```python
from build123d import *

# Parameters (mm, degrees)
SKETCH1_W                = 170
SKETCH1_H                = 45
BOSS_EXTRUDE1_DEPTH      = 3
SKETCH2_W                = 6
SKETCH2_H                = 3
BOSS_EXTRUDE2_DEPTH      = 3
LPATTERN1_COUNT          = 7
LPATTERN1_PITCH          = 12
LPATTERN1_COL_COUNT      = 8
LPATTERN1_COL_PITCH      = 12
SKETCH3_W                = 6
SKETCH3_H                = 3
BOSS_EXTRUDE3_DEPTH      = 3
LPATTERN2_COUNT          = 2
LPATTERN2_PITCH          = 12
LPATTERN2_COL_COUNT      = 3
LPATTERN2_COL_PITCH      = 12
MIRROR1_COPY_1_SKETCH_W  = 6
MIRROR1_COPY_1_SKETCH_H  = 3
MIRROR1_COPY_1_DEPTH     = 3
MIRROR1_COPY_2_SKETCH_W  = 6
MIRROR1_COPY_2_SKETCH_H  = 3
MIRROR1_COPY_2_DEPTH     = 3
MIRROR1_COPY_3_SKETCH_W  = 6
MIRROR1_COPY_3_SKETCH_H  = 3
MIRROR1_COPY_3_DEPTH     = 3
MIRROR1_COPY_4_SKETCH_W  = 6
MIRROR1_COPY_4_SKETCH_H  = 3
MIRROR1_COPY_4_DEPTH     = 3
MIRROR1_COPY_5_SKETCH_W  = 6
MIRROR1_COPY_5_SKETCH_H  = 3
MIRROR1_COPY_5_DEPTH     = 3
MIRROR1_COPY_6_SKETCH_W  = 6
MIRROR1_COPY_6_SKETCH_H  = 3
MIRROR1_COPY_6_DEPTH     = 3
MIRROR1_COPY_7_SKETCH_W  = 6
MIRROR1_COPY_7_SKETCH_H  = 3
MIRROR1_COPY_7_DEPTH     = 3
MIRROR1_COPY_8_SKETCH_W  = 6
MIRROR1_COPY_8_SKETCH_H  = 3
MIRROR1_COPY_8_DEPTH     = 3
MIRROR1_COPY_9_SKETCH_W  = 6
MIRROR1_COPY_9_SKETCH_H  = 3
MIRROR1_COPY_9_DEPTH     = 3
MIRROR1_COPY_10_SKETCH_W = 6
MIRROR1_COPY_10_SKETCH_H = 3
MIRROR1_COPY_10_DEPTH    = 3
MIRROR1_COPY_11_SKETCH_W = 6
MIRROR1_COPY_11_SKETCH_H = 3
MIRROR1_COPY_11_DEPTH    = 3
MIRROR1_COPY_12_SKETCH_W = 6
MIRROR1_COPY_12_SKETCH_H = 3
MIRROR1_COPY_12_DEPTH    = 3
MIRROR1_COPY_13_SKETCH_W = 6
MIRROR1_COPY_13_SKETCH_H = 3
MIRROR1_COPY_13_DEPTH    = 3
MIRROR2_COPY_1_SKETCH_W  = 6
MIRROR2_COPY_1_SKETCH_H  = 3
MIRROR2_COPY_1_DEPTH     = 3
MIRROR2_COPY_2_SKETCH_W  = 6
MIRROR2_COPY_2_SKETCH_H  = 3
MIRROR2_COPY_2_DEPTH     = 3
MIRROR2_COPY_3_SKETCH_W  = 6
MIRROR2_COPY_3_SKETCH_H  = 3
MIRROR2_COPY_3_DEPTH     = 3


with BuildPart() as part:
    # Sketch1 → Boss-Extrude1 (new body)
    with BuildSketch(Plane(origin=(0, 0, 0), x_dir=(1, 0, 0), z_dir=(0, 1, 0))):
        Rectangle(SKETCH1_W, SKETCH1_H)
    extrude(amount=BOSS_EXTRUDE1_DEPTH)

    # Sketch2 → Boss-Extrude2 (add)
    with BuildSketch(Plane.XY.offset(22.5)):
        with Locations((6, 1.5)):
            Rectangle(SKETCH2_W, SKETCH2_H)
    boss_extrude2 = extrude(amount=BOSS_EXTRUDE2_DEPTH)

    # LPattern1: Boss-Extrude2 ×7
    with Locations(*[(i * LPATTERN1_PITCH, 0, 0) for i in range(1, LPATTERN1_COUNT)]):
        add(boss_extrude2)

    # LPattern1 col: Boss-Extrude2 ×8
    with Locations(*[(-i * LPATTERN1_COL_PITCH, 0, 0) for i in range(1, LPATTERN1_COL_COUNT)]):
        add(boss_extrude2)

    # Sketch3 → Boss-Extrude3 (add)
    with BuildSketch(Plane(origin=(85, 0, 0), x_dir=(0, 0, -1), z_dir=(1, 0, 0))):
        with Locations((6, 1.5)):
            Rectangle(SKETCH3_W, SKETCH3_H)
    boss_extrude3 = extrude(amount=BOSS_EXTRUDE3_DEPTH)

    # LPattern2: Boss-Extrude3 ×2
    with Locations(*[(0, 0, -i * LPATTERN2_PITCH) for i in range(1, LPATTERN2_COUNT)]):
        add(boss_extrude3)

    # LPattern2 col: Boss-Extrude3 ×3
    with Locations(*[(0, 0, i * LPATTERN2_COL_PITCH) for i in range(1, LPATTERN2_COL_COUNT)]):
        add(boss_extrude3)

    # Mirror1: Boss-Extrude2 across plane
    add(boss_extrude2.mirror(Plane(origin=(0, 0, 0), x_dir=(1, 0, 0), z_dir=(0, 0, -1))))

    # Mirror1 copy 1 sketch → Mirror1 copy 1 (add)
    with BuildSketch(Plane(origin=(12, 0, -22.5), x_dir=(1, 0, 0), z_dir=(0, 0, -1))):
        with Locations((6, -1.5)):
            Rectangle(MIRROR1_COPY_1_SKETCH_W, MIRROR1_COPY_1_SKETCH_H)
    extrude(amount=MIRROR1_COPY_1_DEPTH)

    # Mirror1 copy 2 sketch → Mirror1 copy 2 (add)
    with BuildSketch(Plane(origin=(24, 0, -22.5), x_dir=(1, 0, 0), z_dir=(0, 0, -1))):
        with Locations((6, -1.5)):
            Rectangle(MIRROR1_COPY_2_SKETCH_W, MIRROR1_COPY_2_SKETCH_H)
    extrude(amount=MIRROR1_COPY_2_DEPTH)

    # Mirror1 copy 3 sketch → Mirror1 copy 3 (add)
    with BuildSketch(Plane(origin=(36, 0, -22.5), x_dir=(1, 0, 0), z_dir=(0, 0, -1))):
        with Locations((6, -1.5)):
            Rectangle(MIRROR1_COPY_3_SKETCH_W, MIRROR1_COPY_3_SKETCH_H)
    extrude(amount=MIRROR1_COPY_3_DEPTH)

    # Mirror1 copy 4 sketch → Mirror1 copy 4 (add)
    with BuildSketch(Plane(origin=(48, 0, -22.5), x_dir=(1, 0, 0), z_dir=(0, 0, -1))):
        with Locations((6, -1.5)):
            Rectangle(MIRROR1_COPY_4_SKETCH_W, MIRROR1_COPY_4_SKETCH_H)
    extrude(amount=MIRROR1_COPY_4_DEPTH)

    # Mirror1 copy 5 sketch → Mirror1 copy 5 (add)
    with BuildSketch(Plane(origin=(60, 0, -22.5), x_dir=(1, 0, 0), z_dir=(0, 0, -1))):
        with Locations((6, -1.5)):
            Rectangle(MIRROR1_COPY_5_SKETCH_W, MIRROR1_COPY_5_SKETCH_H)
    extrude(amount=MIRROR1_COPY_5_DEPTH)

    # Mirror1 copy 6 sketch → Mirror1 copy 6 (add)
    with BuildSketch(Plane(origin=(72, 0, -22.5), x_dir=(1, 0, 0), z_dir=(0, 0, -1))):
        with Locations((6, -1.5)):
            Rectangle(MIRROR1_COPY_6_SKETCH_W, MIRROR1_COPY_6_SKETCH_H)
    extrude(amount=MIRROR1_COPY_6_DEPTH)

    # Mirror1 copy 7 sketch → Mirror1 copy 7 (add)
    with BuildSketch(Plane(origin=(-12, 0, -22.5), x_dir=(1, 0, 0), z_dir=(0, 0, -1))):
        with Locations((6, -1.5)):
            Rectangle(MIRROR1_COPY_7_SKETCH_W, MIRROR1_COPY_7_SKETCH_H)
    extrude(amount=MIRROR1_COPY_7_DEPTH)

    # Mirror1 copy 8 sketch → Mirror1 copy 8 (add)
    with BuildSketch(Plane(origin=(-24, 0, -22.5), x_dir=(1, 0, 0), z_dir=(0, 0, -1))):
        with Locations((6, -1.5)):
            Rectangle(MIRROR1_COPY_8_SKETCH_W, MIRROR1_COPY_8_SKETCH_H)
    extrude(amount=MIRROR1_COPY_8_DEPTH)

    # Mirror1 copy 9 sketch → Mirror1 copy 9 (add)
    with BuildSketch(Plane(origin=(-36, 0, -22.5), x_dir=(1, 0, 0), z_dir=(0, 0, -1))):
        with Locations((6, -1.5)):
            Rectangle(MIRROR1_COPY_9_SKETCH_W, MIRROR1_COPY_9_SKETCH_H)
    extrude(amount=MIRROR1_COPY_9_DEPTH)

    # Mirror1 copy 10 sketch → Mirror1 copy 10 (add)
    with BuildSketch(Plane(origin=(-48, 0, -22.5), x_dir=(1, 0, 0), z_dir=(0, 0, -1))):
        with Locations((6, -1.5)):
            Rectangle(MIRROR1_COPY_10_SKETCH_W, MIRROR1_COPY_10_SKETCH_H)
    extrude(amount=MIRROR1_COPY_10_DEPTH)

    # Mirror1 copy 11 sketch → Mirror1 copy 11 (add)
    with BuildSketch(Plane(origin=(-60, 0, -22.5), x_dir=(1, 0, 0), z_dir=(0, 0, -1))):
        with Locations((6, -1.5)):
            Rectangle(MIRROR1_COPY_11_SKETCH_W, MIRROR1_COPY_11_SKETCH_H)
    extrude(amount=MIRROR1_COPY_11_DEPTH)

    # Mirror1 copy 12 sketch → Mirror1 copy 12 (add)
    with BuildSketch(Plane(origin=(-72, 0, -22.5), x_dir=(1, 0, 0), z_dir=(0, 0, -1))):
        with Locations((6, -1.5)):
            Rectangle(MIRROR1_COPY_12_SKETCH_W, MIRROR1_COPY_12_SKETCH_H)
    extrude(amount=MIRROR1_COPY_12_DEPTH)

    # Mirror1 copy 13 sketch → Mirror1 copy 13 (add)
    with BuildSketch(Plane(origin=(-84, 0, -22.5), x_dir=(1, 0, 0), z_dir=(0, 0, -1))):
        with Locations((6, -1.5)):
            Rectangle(MIRROR1_COPY_13_SKETCH_W, MIRROR1_COPY_13_SKETCH_H)
    extrude(amount=MIRROR1_COPY_13_DEPTH)

    # Mirror2: Boss-Extrude3 across plane
    add(boss_extrude3.mirror(Plane.ZY))

    # Mirror2 copy 1 sketch → Mirror2 copy 1 (add)
    with BuildSketch(Plane(origin=(-85, 0, -12), x_dir=(0, 0, -1), z_dir=(-1, 0, 0))):
        with Locations((6, -1.5)):
            Rectangle(MIRROR2_COPY_1_SKETCH_W, MIRROR2_COPY_1_SKETCH_H)
    extrude(amount=MIRROR2_COPY_1_DEPTH)

    # Mirror2 copy 2 sketch → Mirror2 copy 2 (add)
    with BuildSketch(Plane(origin=(-85, 0, 12), x_dir=(0, 0, -1), z_dir=(-1, 0, 0))):
        with Locations((6, -1.5)):
            Rectangle(MIRROR2_COPY_2_SKETCH_W, MIRROR2_COPY_2_SKETCH_H)
    extrude(amount=MIRROR2_COPY_2_DEPTH)

    # Mirror2 copy 3 sketch → Mirror2 copy 3 (add)
    with BuildSketch(Plane(origin=(-85, 0, 24), x_dir=(0, 0, -1), z_dir=(-1, 0, 0))):
        with Locations((6, -1.5)):
            Rectangle(MIRROR2_COPY_3_SKETCH_W, MIRROR2_COPY_3_SKETCH_H)
    extrude(amount=MIRROR2_COPY_3_DEPTH)


solid = part.part
```
Model file for the job. Use its own axes, mm. A direction names the side the tool comes from. Coordinates: 2 decimals unless noted, no trailing zeros. Loops run counter-clockwise (first coordinate to the right, second up) from the corner with the lowest first, then second, coordinate; pieces in that order, holes last. Notation, with made-up numbers: (57, -25) - (109, -25) arc R32 cw to (109, 1) - close; hole circle Ø8 at (-33.5, 77.5). An arc over 180 degrees is marked (long way). Write item = value, one per line. Start each with the question number.
Item 1: 3-axis set-ups, long thin cutter, end or side, ignore diameter. For faces 5 (the face through (-83, 1, -22.5)), 6 (the face through (15, 1, 24)), 7 (the face through (0, 1, -22.5)), 8 (the face through (-86, 1, -9)), 9 (the face through (78, 2, 25.5)): which of +Z, -Z, +X, -X, +Y, -Y reach the whole face in a straight line?
Item 2: Saw through at B-B, the plane z = -12. List the corners of the cut face in (x, y).
Item 3: Wall check: probe 1 along Z at (x, y) = (25.5, 1.05); probe 2 along X at (y, z) = (2.6, -10.5). Give the ranges that are in metal, low to high. Write a range as [from, to].
Item 4: Pull direction X, two halves, no side cores. Call faces 1 (the face through (88, 2, 18)), 2 (the face through (42, 2, 25.5)), 3 (the face through (24, 1, -22.5)), 4 (the face through (-9, 1, 24)): +X half, -X half, draft (parallel to the pull), parting line (faces both ways), or undercut.
Item 5: Drop flat-ended pins along their axis: pin 1 Ø0.9 at (x, y) = (36.5, 2) entering from -Z; pin 2 Ø1.5 at (y, z) = (1.5, -24.5) entering from -X; pin 3 Ø1.5 at (x, y) = (58.5, 1) entering from +Z. Give the stop position or say it passes through.
Item 6: Saw through at A-A, the plane x = -59.5. List the corners of the cut face in (y, z), then the cut area to 3 significant figures.
Answers:
q1.face_5 = -Z, -X, +Y, -Y
q1.face_6 = +Z, +Y, -Y
q1.face_7 = -Z, +Y, -Y
q1.face_8 = -X, +Y, -Y
q1.face_9 = +Z, +X, -X, +Y, -Y
q2.outline = (-85, 0) - (85, 0) - (85, 3) - (-85, 3) - close
q3.probe_1 = [-22.5, 22.5]
q3.probe_2 = [-85, 85]
q4.face_1 = +X half
q4.face_2 = draft
q4.face_3 = undercut
q4.face_4 = undercut
q5.pin_1 = -22.5
q5.pin_2 = -81
q5.pin_3 = 22.5
q6.outline = (0, -22.5) - (3, -22.5) - (3, 22.5) - (0, 22.5) - close
q6.area = 135 mm2
